Verification items for the finished model (mm, model axes). Face numbers are marked on the shaded views. A direction names the side the tool comes from. Round coordinates to 2 decimals unless told otherwise and drop trailing zeros. Write each loop counter-clockwise with the first axis right and the second up, starting at its lowest first coordinate (ties: lowest second). Pieces come first, ordered by that corner, then holes. Notation, with made-up numbers: (69.5, 44.5) - (76.5, 44.5) arc R21 cw to (76.5, 68.5) - close; hole circle Ø4 at (-29.5, 45). An arc over 180 degrees is marked (long way). Answer as a JSON object with one key per item and string values. Group by question number.
1) Mould release check, pull along Z, two halves, no side actions. Record for the marked faces 1, 2 and 3: +Z half, -Z half, draft (parallel to the pull), parting line (faces both ways), or undercut.
2) Thickness scan on line 1 (X direction, y = -33, z = 26); line 2 (Z direction, x = 61.5, y = -31); line 3 (Y direction, x = 54, z = 7.5) (3 decimals). Record the ranges inside material, lowest first.
3) Go/stop test with flat-tipped pins: pin 1 Ø5 at (x, z) = (-22.225, -22.225) entering from -Y (3 decimals); pin 2 Ø4 at (y, z) = (-14, -13.5) entering from -X; pin 3 Ø2 at (x, y) = (23.5, -14.5) entering from +Z; pin 4 Ø12 at (x, y) = (-5, -15) entering from -Z. Record where each tip stops, or that it passes through.
4) Section check B-B (x = -31.5). State how many separate pieces and enclosed holes the cut face has, then the cut area to 3 significant figures.
5) Set-up check for the marked faces 4, 5, 6 and 7: record each of +Z, -Z, +X, -X, +Y, -Y from which the full face is reachable in a straight line by a thin tool's end or side.
6) Section check A-A (z = 0). Enter the section's corners in (x, y) (3 decimals).
```python
from build123d import *

# Parameters (mm, degrees)
BOSS_EXTRU_1_DEPTH                              = 31.75
CONG_1_R                                        = 6.35
CONG_2_R                                        = 3.175
ESQUISSE4_R                                     = 7.14375
ESQUISSE4_R_2                                   = 2.2225
ENL_V_MAT_EXTRU_1_DEPTH                         = 105.582398734
CHAMBRAGE_POUR_VIS_T_TE_CYLINDRIQUE_D           = 3.4544
CHAMBRAGE_POUR_VIS_T_TE_CYLINDRIQUE_DEPTH       = 3.175
CHAMBRAGE_POUR_VIS_T_TE_CYLINDRIQUE_CBORE_D     = 6.35
CHAMBRAGE_POUR_VIS_T_TE_CYLINDRIQUE_CBORE_DEPTH = 1.5875
R_P_T_START                                     = -75.40625
R_P_T_PAR_COURBE1_OUTLINE_R                     = 3.175
R_P_T_PAR_COURBE1_DEPTH                         = 1.5875
R_P_T_START_2                                   = -73.81875
R_P_T_PAR_COURBE1_2_OUTLINE_R                   = 1.7272
R_P_T_PAR_COURBE1_2_DEPTH                       = 1.5875
ENL_V_MAT_EXTRU_4_REACH                         = 173.907
BOSS_EXTRU_2_START                              = -3.175
BOSS_EXTRU_2_DEPTH                              = 3.175
CONG_3_R                                        = 1.5875
CONG_3_OF_SYM_TRIE2_R                           = 1.5875
CONG_4_R                                        = 3.175


# Read off the part's stored shape, not the designer's step: Répét. par courbe1
with BuildPart() as part:
    # Esquisse3 → Boss.-Extru.1 (new, symmetric)
    with BuildSketch(Plane.XY):
        Polygon((-75.40625, 0), (75.40625, 0), (75.40625, -47.625), (85.725, -47.625), (85.725, -50.8), (72.23125, -50.8), (72.23125, -3.175), (-72.23125, -3.175), (-72.23125, -50.8), (-85.725, -50.8), (-85.725, -47.625), (-75.40625, -47.625), align=None)
    extrude(amount=BOSS_EXTRU_1_DEPTH, both=True)

    # Congé1
    cong_1_edges = [part.edges().sort_by_distance(p)[0] for p in [
        (72.23125, -50.8, 0),
        (-72.23125, -50.8, 0),
        (-75.40625, 0, 0),
        (75.40625, 0, 0),
    ]]
    fillet(cong_1_edges, radius=CONG_1_R)

    # Congé2
    cong_2_edges = [part.edges().sort_by_distance(p)[0] for p in [
        (75.40625, -47.625, 0),
        (72.23125, -3.175, 0),
        (-72.23125, -3.175, 0),
        (-75.40625, -47.625, 0),
    ]]
    fillet(cong_2_edges, radius=CONG_2_R)

    # Esquisse4 → Enlèv. mat.-Extru.1 (cut, through all)
    with BuildSketch(Plane(origin=(0, 0, 0), x_dir=(1, 0, 0), z_dir=(0, 1, 0))):
        with Locations(Location((-34.925, -19.05, 0), (0, 0, 270))):
            Circle(ESQUISSE4_R)
        with Locations(Location((-22.225, -22.225, 0), (0, 0, 270))):
            Circle(ESQUISSE4_R_2)
        with Locations(Location((22.225, -22.225, 0), (0, 0, 270))):
            Circle(ESQUISSE4_R_2)
        with Locations(Location((34.925, -19.05, 0), (0, 0, 270))):
            Circle(ESQUISSE4_R)
        with Locations(Location((22.225, 22.225, 0), (0, 0, 270))):
            Circle(ESQUISSE4_R_2)
        with Locations(Location((-22.225, 22.225, 0), (0, 0, 270))):
            Circle(ESQUISSE4_R_2)
    extrude(amount=-ENL_V_MAT_EXTRU_1_DEPTH, mode=Mode.SUBTRACT)

    # Chambrage pour vis à tête cylindrique à 6 pans creux (vis CHC) #54
    with Locations(Plane.ZY.offset(75.40625)):
        with Locations((-15.494, -27.1018)):
            chambrage_pour_vis_t_te_cylindrique = CounterBoreHole(CHAMBRAGE_POUR_VIS_T_TE_CYLINDRIQUE_D / 2, CHAMBRAGE_POUR_VIS_T_TE_CYLINDRIQUE_CBORE_D / 2, CHAMBRAGE_POUR_VIS_T_TE_CYLINDRIQUE_CBORE_DEPTH, depth=CHAMBRAGE_POUR_VIS_T_TE_CYLINDRIQUE_DEPTH)

    # Répét. par courbe1 outline → Répét. par courbe1 (cut)
    with BuildSketch(Plane.YZ.offset(R_P_T_START)):
        with Locations((-40.519997606, -7.747)):
            Circle(R_P_T_PAR_COURBE1_OUTLINE_R)
        with Locations((-40.519997606, 7.747)):
            Circle(R_P_T_PAR_COURBE1_OUTLINE_R)
        with Locations((-27.1018, 15.494)):
            Circle(R_P_T_PAR_COURBE1_OUTLINE_R)
        with Locations((-13.683602394, 7.747)):
            Circle(R_P_T_PAR_COURBE1_OUTLINE_R)
        with Locations((-13.683602394, -7.747)):
            Circle(R_P_T_PAR_COURBE1_OUTLINE_R)
    r_p_t_par_courbe1 = extrude(amount=R_P_T_PAR_COURBE1_DEPTH, mode=Mode.SUBTRACT)

    # R_p_t. par courbe1 2 outline → R_p_t. par courbe1 2 (cut)
    with BuildSketch(Plane.YZ.offset(R_P_T_START_2)):
        with Locations((-40.519997606, -7.747)):
            Circle(R_P_T_PAR_COURBE1_2_OUTLINE_R)
        with Locations((-40.519997606, 7.747)):
            Circle(R_P_T_PAR_COURBE1_2_OUTLINE_R)
        with Locations((-27.1018, 15.494)):
            Circle(R_P_T_PAR_COURBE1_2_OUTLINE_R)
        with Locations((-13.683602394, 7.747)):
            Circle(R_P_T_PAR_COURBE1_2_OUTLINE_R)
        with Locations((-13.683602394, -7.747)):
            Circle(R_P_T_PAR_COURBE1_2_OUTLINE_R)
    r_p_t_par_courbe1_2 = extrude(amount=R_P_T_PAR_COURBE1_2_DEPTH, mode=Mode.SUBTRACT)

    # Esquisse6 → Enlèv. mat.-Extru.4 (cut, up to next)
    with BuildSketch(Plane.ZY.offset(75.40625), mode=Mode.PRIVATE) as enl_v_mat_extru_4_sk1:
        with BuildLine():
            Line((6.35, -21.4122), (6.35, -34.1122))
            ThreePointArc((6.35, -34.1122), (0, -40.4622), (-6.35, -34.1122))
            Line((-6.35, -34.1122), (-6.35, -21.4122))
            ThreePointArc((-6.35, -21.4122), (0, -15.0622), (6.35, -21.4122))
        make_face()
    enl_v_mat_extru_4_tool1 = extrude(enl_v_mat_extru_4_sk1.sketch, amount=-ENL_V_MAT_EXTRU_4_REACH, mode=Mode.PRIVATE) & part.part
    enl_v_mat_extru_4 = enl_v_mat_extru_4_tool1.solids().sort_by_distance((-75.40625, -27.7622, 0))[0]
    add(enl_v_mat_extru_4, mode=Mode.SUBTRACT)

    # Symétrie1: Chambrage pour vis à tête cylindrique à 6 pans creux (vis CHC) #54, Répét. par courbe1, R_p_t. par courbe1 2, Enlèv. mat.-Extru.4 across plane
    add(chambrage_pour_vis_t_te_cylindrique.mirror(Plane(origin=(0, 0, 0), x_dir=(0, 0, 1), z_dir=(1, 0, 0))), mode=Mode.SUBTRACT)
    add(r_p_t_par_courbe1.mirror(Plane(origin=(0, 0, 0), x_dir=(0, 0, 1), z_dir=(1, 0, 0))), mode=Mode.SUBTRACT)
    add(r_p_t_par_courbe1_2.mirror(Plane(origin=(0, 0, 0), x_dir=(0, 0, 1), z_dir=(1, 0, 0))), mode=Mode.SUBTRACT)
    add(enl_v_mat_extru_4.mirror(Plane(origin=(0, 0, 0), x_dir=(0, 0, 1), z_dir=(1, 0, 0))), mode=Mode.SUBTRACT)

    # Esquisse26 → Boss.-Extru.2 (add)
    with BuildSketch(Plane.XY.offset(30.1625).offset(BOSS_EXTRU_2_START)):
        with BuildLine():
            Line((-15.875, -10.60369343), (-72.23125, -43.140989538))
            Line((-72.23125, -43.140989538), (-72.23125, -6.35))
            ThreePointArc((-72.23125, -6.35), (-71.30131403, -4.10493597), (-69.05625, -3.175))
            Line((-69.05625, -3.175), (69.05625, -3.175))
            ThreePointArc((69.05625, -3.175), (71.30131403, -4.10493597), (72.23125, -6.35))
            Line((72.23125, -6.35), (72.23125, -43.140989538))
            Line((72.23125, -43.140989538), (15.875, -10.60369343))
            ThreePointArc((15.875, -10.60369343), (0, -6.35), (-15.875, -10.60369343))
        make_face()
        Polygon((-69.05625, -6.35), (-21.20738686, -6.35), (-69.05625, -33.975554014), align=None, mode=Mode.SUBTRACT)
        Polygon((21.20738686, -6.35), (69.05625, -33.975554014), (69.05625, -6.35), align=None, mode=Mode.SUBTRACT)
    boss_extru_2 = extrude(amount=BOSS_EXTRU_2_DEPTH)

    # Congé3
    cong_3_edges = [part.edges().sort_by_distance(p)[0] for p in [
        (-69.05625, -6.35, 28.575),
        (-21.20738686, -6.35, 28.575),
        (-69.05625, -33.975554014, 28.575),
        (69.05625, -6.35, 28.575),
        (69.05625, -33.975554014, 28.575),
        (21.20738686, -6.35, 28.575),
    ]]
    fillet(cong_3_edges, radius=CONG_3_R)

    # Symétrie2: Boss.-Extru.2 across plane
    add(boss_extru_2.mirror(Plane.XY))

    # Congé3 of Symétrie2
    cong_3_of_sym_trie2_edges = [part.edges().sort_by_distance(p)[0] for p in [
        (-69.05625, -6.35, -28.575),
        (-21.20738686, -6.35, -28.575),
        (-69.05625, -33.975554014, -28.575),
        (69.05625, -6.35, -28.575),
        (69.05625, -33.975554014, -28.575),
        (21.20738686, -6.35, -28.575),
    ]]
    fillet(cong_3_of_sym_trie2_edges, radius=CONG_3_OF_SYM_TRIE2_R)

    # Congé4
    # the kernel refuses this fillet: 3.175 mm, written as the material it adds along each edge
    with BuildSketch(Plane(origin=(-72.23125, -43.140989538, 26.9875), x_dir=(-0.005971670671685116, -0.9999821694157295, 0), z_dir=(0, 0, 1)), Plane(origin=(72.23125, -43.140989538, -26.9875), x_dir=(0.0059716706716850905, -0.9999821694157296, 0), z_dir=(0, 0, -1))) as cong_4_piece_1:
        with BuildLine():
            CenterArc((1.822789642, 3.171034898), CONG_4_R, 210.34215356, 56.794076382)
            Line((-0.91731196, 1.567143316), (-1.191322121, 1.406754157))
            Line((-1.191322121, 1.406754157), (-0.27401016, -0.160389158))
            Line((-0.27401016, -0.160389158), (0.001896005, -0.317494339))
            ThreePointArc((0.001896005, -0.317494339), (1.310883127, -0.309677359), (1.648299424, -0.31710349))
            Line((1.648299424, -0.31710349), (1.664162171, 0))
        make_face()
    extrude(amount=3.175)
    with BuildSketch(Plane(origin=(72.23125, -43.140989538, 26.9875), x_dir=(0.0059716706716850905, -0.9999821694157296, 0), z_dir=(0, 0, 1))) as cong_4_piece_2:
        with BuildLine():
            CenterArc((1.822789642, -3.171034898), CONG_4_R, 92.863770058, 56.794076382)
            Line((-0.91731196, -1.567143316), (-1.191322121, -1.406754157))
            Line((-1.191322121, -1.406754157), (-0.27401016, 0.160389158))
            Line((-0.27401016, 0.160389158), (0.001896005, 0.317494339))
            ThreePointArc((0.001896005, 0.317494339), (1.310883127, 0.309677359), (1.648299424, 0.31710349))
            Line((1.648299424, 0.31710349), (1.664162171, 0))
        make_face()
    extrude(amount=3.175)
    with BuildSketch(Plane(origin=(-72.23125, -43.140989538, -26.9875), x_dir=(0.8660254037844383, 0.5000000000000007, 0), z_dir=(0, 0, -1))) as cong_4_piece_3:
        with BuildLine():
            CenterArc((1.815874281, 3.175), CONG_4_R, 213.205923618, 56.794076382)
            Line((-0.840672661, 1.436212105), (-1.106327355, 1.262333315))
            ThreePointArc((-1.106327355, 1.262333315), (-0.929468297, 0.974886314), (-0.274963066, -0.15875))
            Line((-0.274963066, -0.15875), (0, -0.3175))
            Line((0, -0.3175), (1.815874281, -0.3175))
            Line((1.815874281, -0.3175), (1.815874281, 0))
        make_face()
    extrude(amount=3.175)


solid = part.part
```
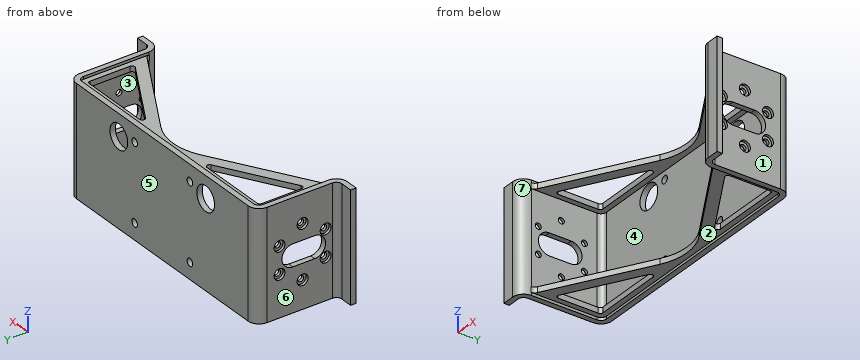
Returned:
{
 "1": {"face 1": "draft", "face 2": "-Z half", "face 3": "undercut"},
 "2": {"line 1": "-75.41 to -72.23, 72.23 to 75.41", "line 2": "-30.16 to -26.99, 26.99 to 30.16", "line 3": "-3.175 to 0"},
 "3": {"pin 1": "y = -3.175", "pin 2": "x = -75.41", "pin 3": "z = 30.16", "pin 4": "through"},
 "4": {"separate pieces": "4", "enclosed holes": "0", "area": "229 mm2"},
 "5": {"face 4": "-Y", "face 5": "+Z, -Z, +X, -X, +Y", "face 6": "+Z, -Z, -X, +Y", "face 7": "+Z, -Z, -Y"},
 "6": {"outline": "(-85.725, -50.8) - (-78.581, -50.8) arc R6.35 ccw to (-72.231, -44.45) - (-72.231, -40.462) - (-75.406, -40.462) - (-75.406, -44.45) arc R3.175 cw to (-78.581, -47.625) - (-85.725, -47.625) - close; (-75.406, -15.062) - (-72.231, -15.062) - (-72.231, -6.35) arc R3.175 cw to (-69.056, -3.175) - (69.056, -3.175) arc R3.175 cw to (72.231, -6.35) - (72.231, -15.062) - (75.406, -15.062) - (75.406, -6.35) arc R6.35 ccw to (69.056, 0) - (-69.056, 0) arc R6.35 ccw to (-75.406, -6.35) - close; (72.231, -44.45) arc R6.35 ccw to (78.581, -50.8) - (85.725, -50.8) - (85.725, -47.625) - (78.581, -47.625) arc R3.175 cw to (75.406, -44.45) - (75.406, -40.462) - (72.231, -40.462) - close"}
}
